Work out the finished part from the listing and answer in its coordinate system (mm). Face numbers are marked on the shaded views. A direction names the side the tool comes from. Round coordinates to 2 decimals unless told otherwise and drop trailing zeros. Answer as CSV lines item,"result". Start each with the question number.
```python
from build123d import *

# Parameters (mm, degrees)
SKETCH001_R             = 3
PAD_DEPTH               = 29
BODY001_PLACEMENT_ANGLE = 34
REVOLUTION_ANGLE        = -180
CHAMFER_SIZE            = 1


with BuildPart() as body001:
    # Sketch001 → Pad (new body)
    with BuildSketch(Plane.XZ):
        Circle(SKETCH001_R)
    extrude(amount=-PAD_DEPTH)


with BuildPart() as body001_1:
    # Body001 placement: moved
    add(body001.part.moved(Location((7, -3, 0))).rotate(Axis((7, -3, 0), (0, 0, 1)), BODY001_PLACEMENT_ANGLE))


with BuildPart() as body:
    # Sketch → Revolution (revolve)
    with BuildSketch(Plane.XY):
        with BuildLine():
            Line((9.5, 15), (12.5, 15))
            ThreePointArc((12.5, 15), (11.62132, 17.12132), (9.5, 18))
            Line((0, 18), (9.5, 18))
            Line((0, 0), (0, 18))
            Line((0, 0), (7.5, 0))
            ThreePointArc((7.5, 0), (8.914214, 0.585786), (9.5, 2))
            Line((9.5, 15), (9.5, 2))
        make_face()
    revolve(axis=Axis((0, 0, 0), (0, 1, 0)), revolution_arc=REVOLUTION_ANGLE)

    # Boolean: cut Body001
    add(body001_1.part, mode=Mode.SUBTRACT)

    # Chamfer
    chamfer_edges = [body.edges().sort_by_distance(p)[0] for p in [
        (-5.63609, 18, 2.719202),
        (3.511353, 0, 2.743109),
    ]]
    chamfer(chamfer_edges, length=CHAMFER_SIZE)


solid = body.part
```
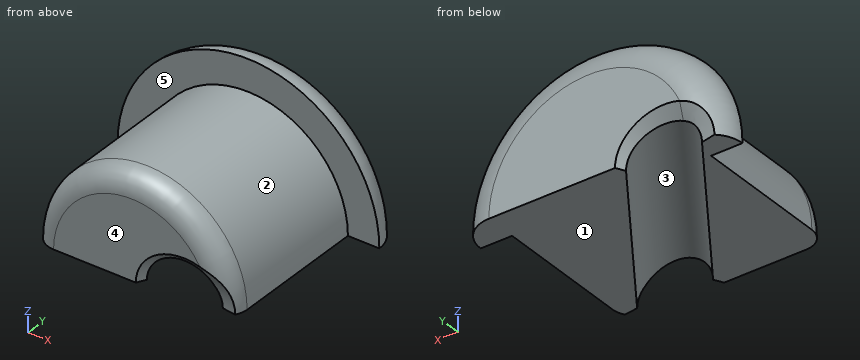
Item 1: Determine the mould class of the marked faces 1, 2 and 3 for opening direction X: pulls with the +X half, pulls with the -X half, needs draft (parallel to the pull), parting line crosses it, or undercut.
Item 2: Flat-ended cylindrical pins translate along their axes: pin 1 Ø3 at (y, z) = (6.5, 3) entering from -X; pin 2 Ø1.5 at (y, z) = (5, 4.5) entering from +X; pin 3 Ø1 at (y, z) = (9, 7.5) entering from -X. Find the tip coordinate at first contact, or state that the pin passes through.
Item 3: Find the intervals of material crossed by L1, parallel to X at y = 5, z = 1.75; L2, parallel to Y at x = -5, z = 7.25; L3, parallel to X at y = 11.75, z = 2, in increasing order.
Item 4: Which of the six approach directions +Z, -Z, +X, -X, +Y, -Y give full straight-line access (tool end or side, diameter ignored) to the marked faces 4 and 5?
Answer:
1,face 1,"needs draft"
1,face 2,"parting line crosses it"
1,face 3,"undercut"
2,pin 1,"stops at x = -9.38"
2,pin 2,"stops at x = 8.73"
2,pin 3,"stops at x = -6.42"
3,L1,"x = -9.34 to -1.34, 4.54 to 9.34"
3,L2,"y = 0.49 to 18"
3,L3,"x = -9.29 to -5.65, -0.25 to 9.29"
4,face 4,"+Z, -Z, +X, -X, -Y"
4,face 5,"+Z, -Y"
